```python
from build123d import *

# Parameters (mm, degrees)
F0_R     = 75.686993118
F1_DEPTH = 25.4
F2_DEPTH = 25.4
F7_R     = 51.508951791
F8_DEPTH = 50.801


# Not quite as in the source:
# - a feature of the source that left no trace in its solid (it failed there, or was rolled back) is left out
# - the program builds the solid bodies; features that only make, move or delete a surface that nothing else refers to are left out


with BuildPart() as f1:
    # F0 (on Top) → F1 (new body)
    with BuildSketch(Plane.XY):
        Circle(F0_R)
    extrude(amount=F1_DEPTH)

    # F2 (add): a face of the model
    f2_faces = [f1.faces().sort_by_distance(p)[0] for p in [
        (0, 0, 0),
    ]]
    extrude(f2_faces, amount=F2_DEPTH)

    # F7 (on face) → F8 (cut, through all)
    with BuildSketch(Plane(origin=(0, 0, -25.4), x_dir=(1, 0, 0), z_dir=(0, 0, -1))):
        Circle(F7_R)
    extrude(amount=-F8_DEPTH, mode=Mode.SUBTRACT)


solid = f1.part
```
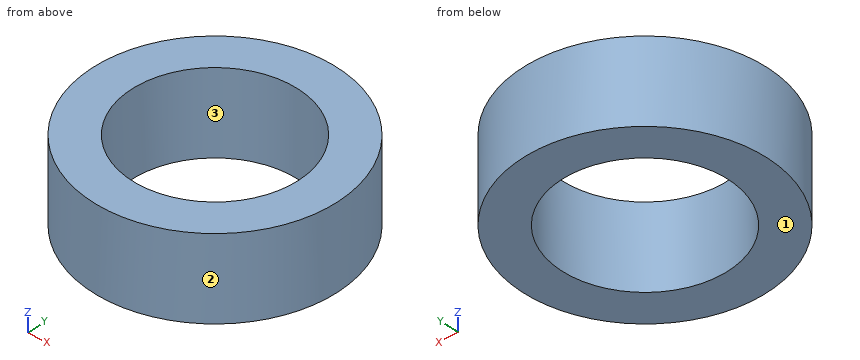
The listing builds one solid part. Answer for the finished solid, in the listing's coordinates (mm). Face numbers are marked on the shaded views. Coordinates: 2 decimals unless noted, no trailing zeros. Write each loop counter-clockwise with the first axis right and the second up, starting at its lowest first coordinate (ties: lowest second). Pieces come first, ordered by that corner, then holes. Notation, with made-up numbers: (10.5, 7.25) - (36.5, 7.25) arc R27 cw to (36.5, 45.25) - close; hole circle Ø11 at (65.25, 12). An arc over 180 degrees is marked (long way). Return JSON: item names as keys, results as strings. Group by question number.
1. A cutting plane is placed at A-A, the plane y = 0. Determine the outline of the cut face in (x, z).
2. Determine the mould class of the marked faces 1, 2 and 3 for opening direction Y: released by +Y, released by -Y, zero draft, split by the parting line, or undercut.
3. A cutting plane is placed at D-D, the plane x = -58.5. Determine the outline of the cut face in (y, z), plus the area to 3 significant figures.
4. A cutting plane is placed at C-C, the plane z = -0.5. Determine the outline of the cut face in (x, y), plus the area to 3 significant figures.
5. Straight lines are drawn through the part: L1, parallel to Y at x = 0, z = 4; L2, parallel to X at y = -41, z = -9; L3, parallel to X at y = -2.5, z = -8. For each, find the intervals that lie inside material, in ascending order.
6. Given pin 1 (6 mm diameter, centred on x = -43.5, z = -0.5, fed in from +Y); pin 2 (10 mm diameter, centred on x = -53.5, z = -2.5, fed in from -Y); pin 3 (6 mm diameter, centred on y = -37, z = 12, fed in from +X), each flat-ended and moving along its own axis, determine where each tip first touches the part or whether it passes through.
Ans:
{
 "1": {"outline": "(-75.69, -25.4) - (-51.51, -25.4) - (-51.51, 25.4) - (-75.69, 25.4) - close; (51.51, -25.4) - (75.69, -25.4) - (75.69, 25.4) - (51.51, 25.4) - close"},
 "2": {"face 1": "zero draft", "face 2": "split by the parting line", "face 3": "undercut"},
 "3": {"outline": "(-48.02, -25.4) - (48.02, -25.4) - (48.02, 25.4) - (-48.02, 25.4) - close", "area": "4,880 mm²"},
 "4": {"outline": "circle Ø151.37 at (0, 0); hole circle Ø103.02 at (0, 0)", "area": "9,660 mm²"},
 "5": {"L1": "-75.69 to -51.51, 51.51 to 75.69", "L2": "-63.62 to -31.18, 31.18 to 63.62", "L3": "-75.65 to -51.45, 51.45 to 75.65"},
 "6": {"pin 1": "y = 63.94", "pin 2": "y = -58.11", "pin 3": "x = 67.62"}
}
